from build123d import *

# Parameters (mm, degrees)
SKETCH1_R            = 76.2
SKETCH1_R_2          = 71.12
BOSS_EXTRUDE8_DEPTH  = 25.4
SKETCH1_3_R          = 2.652133243
BOSS_EXTRUDE9_DEPTH  = 6.35
SKETCH1_4_R          = 4.7625
BOSS_EXTRUDE10_DEPTH = 9.525
CIRPATTERN2_COUNT    = 3


with BuildPart() as part:
    # Sketch1 → Boss-Extrude8 (new, symmetric)
    with BuildSketch(Plane.XY):
        Circle(SKETCH1_R)
        Circle(SKETCH1_R_2, mode=Mode.SUBTRACT)
    extrude(amount=BOSS_EXTRUDE8_DEPTH, both=True)

    # Sketch1_3 → Boss-Extrude9 (add)
    # profile 1 of 3: a face of its own
    with BuildSketch(Plane.XY):
        with BuildLine():
            Line((-51.489686485, -12.770329882), (-64.2646615, -30.464859794))
            ThreePointArc((-64.2646615, -30.464859794), (-60.982470201, -36.594982282), (-57.117332526, -42.375284367))
            add(Edge.make_bspline(
                [(-51.489686485, -12.770329882), (-51.760230573, -13.369074965), (-52.951716514, -16.131352485), (-54.800495305, -21.526228156), (-56.429552058, -29.189681258), (-57.070959365, -36.064182845), (-57.141142785, -40.491289733), (-57.121192418, -42.135824786), (-57.117332526, -42.375284367)],
                knots=[0.741105641, 0.741105641, 0.741105641, 0.741105641, 0.756730641, 0.8125, 0.875, 0.9375, 0.96875, 0.974071806, 0.974071806, 0.974071806, 0.974071806], degree=3))
        make_face()
        with Locations((-59.434967194, -31.713129844)):
            Circle(SKETCH1_3_R, mode=Mode.SUBTRACT)
    # profile 2 of 3: a face of its own
    with BuildSketch(Plane.XY):
        with BuildLine():
            ThreePointArc((-57.117332526, -42.375284367), (-55.813104666, -44.078926343), (-54.458080516, -45.74245147))
            add(Edge.make_bspline(
                [(2.569011428, 12.437450715), (-15.538204508, 21.223476417), (-46.586683763, 7.69387074), (-55.93582443, -18.200568272), (-54.458080516, -45.74245147)],
                knots=[0.164688389, 0.164688389, 0.164688389, 0.164688389, 0.164688389, 1, 1, 1, 1, 1], degree=4))
            ThreePointArc((2.569011428, 12.437450715), (9.846736645, 8.020709285), (12.7, 0))
            ThreePointArc((12.7, 0), (12.581598046, -1.730141787), (12.228599905, -3.42802339))
            add(Edge.make_bspline(
                [(15.157020591, 0.643933082), (14.443060628, -2.918429068), (12.228599905, -3.42802339)],
                knots=[0, 0, 0, 0.719883781, 0.719883781, 0.719883781], degree=2))
            add(Edge.make_bspline(
                [(15.157020591, 0.643933082), (14.991425957, 1.275783561), (14.604911637, 2.54097033), (13.667954828, 4.887393309), (12.183192976, 7.556706342), (9.969654094, 10.294956422), (6.534622803, 13.326938907), (1.520056493, 15.963955949), (-5.168911286, 17.446899809), (-12.189081027, 17.436980233), (-21.635438647, 15.634364862), (-33.013454155, 10.343487809), (-43.696960831, 0.683796899), (-49.136108914, -7.765497225), (-51.219142397, -12.1715848), (-51.489686485, -12.770329882)],
                knots=[0, 0, 0, 0, 0.015625, 0.03125, 0.0625, 0.09375, 0.125, 0.1875, 0.25, 0.3125, 0.375, 0.5, 0.625, 0.725480641, 0.741105641, 0.741105641, 0.741105641, 0.741105641], degree=3))
            add(Edge.make_bspline(
                [(-51.489686485, -12.770329882), (-51.760230573, -13.369074965), (-52.951716514, -16.131352485), (-54.800495305, -21.526228156), (-56.429552058, -29.189681258), (-57.070959365, -36.064182845), (-57.141142785, -40.491289733), (-57.121192418, -42.135824786), (-57.117332526, -42.375284367)],
                knots=[0.741105641, 0.741105641, 0.741105641, 0.741105641, 0.756730641, 0.8125, 0.875, 0.9375, 0.96875, 0.974071806, 0.974071806, 0.974071806, 0.974071806], degree=3))
        make_face()
    # profile 3 of 3: a face of its own
    with BuildSketch(Plane.XY):
        with BuildLine():
            ThreePointArc((12.7, 0), (9.846736645, 8.020709285), (2.569011428, 12.437450715))
            add(Edge.make_bspline(
                [(12.7, 0), (11.504351428, 4.56217151), (9.205933773, 8.105542424), (6.138994382, 10.705215229), (2.569011428, 12.437450715)],
                knots=[0, 0, 0, 0, 0, 0.164688389, 0.164688389, 0.164688389, 0.164688389, 0.164688389], degree=4))
        make_face()
    boss_extrude9 = extrude(amount=BOSS_EXTRUDE9_DEPTH)

    # Sketch1_4 → Boss-Extrude10 (add, symmetric)
    with BuildSketch(Plane.XY):
        with BuildLine():
            add(Edge.make_bspline(
                [(12.7, 0), (11.504351428, 4.56217151), (9.205933773, 8.105542424), (6.138994382, 10.705215229), (2.569011428, 12.437450715)],
                knots=[0, 0, 0, 0, 0, 0.164688389, 0.164688389, 0.164688389, 0.164688389, 0.164688389], degree=4))
            ThreePointArc((2.569011428, 12.437450715), (-10.847609987, -6.604495254), (12.228599905, -3.42802339))
            ThreePointArc((12.228599905, -3.42802339), (12.581598046, -1.730141787), (12.7, 0))
        make_face()
        with Locations(Location((0, 0, 0), (0, 0, 180))):
            Circle(SKETCH1_4_R, mode=Mode.SUBTRACT)
    extrude(amount=BOSS_EXTRUDE10_DEPTH, both=True)

    # CirPattern2: Boss-Extrude9 ×3 about axis
    cirpattern2_axis = Axis((0, 0, -27.94), (0, 0, 1))
    for i in range(1, CIRPATTERN2_COUNT):
        add(boss_extrude9.rotate(cirpattern2_axis, i * 360 / CIRPATTERN2_COUNT))


solid = part.part
CAD build for the part. Positions are in the model's coordinates, mm. A direction names the side the tool comes from. Coordinates: 2 decimals unless noted, no trailing zeros. Write each loop counter-clockwise with the first axis right and the second up, starting at its lowest first coordinate (ties: lowest second). Pieces come first, ordered by that corner, then holes. Notation, with made-up numbers: M 40.5,56.5 L 54.5,56.5 A23 ccw 54.5,95.5 Z; hole C 25,-18.5 d7. An arc over 180 degrees is marked long. Answer as a JSON object with one key per item and string values. Group by question number.
1) Mould opens along X. For faces 1 (the face through (-60.47, -46.367, 0.356)), 2 (the face through (-57.788, -21.494, 3.131)), 3 (the face through (50.4, -50.4, 25.4)) say: +X half, -X half, draft (parallel to the pull), parting line (faces both ways), or undercut.
2) Saw through at A-A (z = 17). Write the cut outline in (x, y).
3) Tool access for faces 4 (the face through (10.28, 60.79, 3.13)), 5 (the face through (-10.1, -7.7, 0.1)), 6 (the face through (23, -36, 0)), 7 (the face through (23, -36, 6.35)), 8 (the face through (50.4, -50.4, -25.4)): list every direction of +Z, -Z, +X, -X, +Y, -Y with a clear straight run to the whole face (end or side of a thin tool).
4) Pin check, flat tips, straight feed: pin 1 Ø12.5 at (x, y) = (3, -4) entering from +Z (3 decimals); pin 2 Ø11 at (x, y) = (-1.5, 19) entering from -Z; pin 3 Ø12 at (x, z) = (-29, 20) entering from -Y. Stop position of each tip, or through.
5) Saw through at B-B (y = 9). Give the number of separate pieces and of enclosed holes in the cut face, plus the area to 3 significant figures.
6) Wall check: line 1 (Y direction, x = 0, z = -6); line 2 (Y direction, x = -19.5, z = 1.5); line 3 (X direction, y = 36, z = 1). Give the ranges that are in metal, low to high. Write a range as from..to.
Values follow:
{
 "1": {"face 1": "parting line", "face 2": "undercut", "face 3": "draft"},
 "2": {"outline": "C 0,0 d152.4; hole C 0,0 d142.24"},
 "3": {"face 4": "+Z, -Z", "face 5": "none", "face 6": "-Z", "face 7": "+Z", "face 8": "-Z, +X, -X, +Y, -Y"},
 "4": {"pin 1": "stops at z = 9.525", "pin 2": "stops at z = 0", "pin 3": "stops at y = -72.65"},
 "5": {"separate pieces": "5", "enclosed holes": "0", "area": "917 mm2"},
 "6": {"line 1": "y = -76.2..-71.12, -12.7..-4.76, 4.76..12.7, 71.12..76.2", "line 2": "y = -73.66..-68.39, 13.16..15.81, 68.39..73.66", "line 3": "x = -67.16..-61.34, 19.62..22.3, 61.34..67.16"}
}
